```python
from build123d import *

# Parameters (mm, degrees)
SALIENTE_EXTRUIR1_DEPTH = 111
SALIENTE_EXTRUIR2_DEPTH = 6
CROQUIS3_W              = 20
CROQUIS3_H              = 5
SALIENTE_EXTRUIR3_DEPTH = 2
SALIENTE_EXTRUIR4_DEPTH = 6
SALIENTE_EXTRUIR5_DEPTH = 2
CROQUIS6_R              = 2
CORTAR_EXTRUIR1_DEPTH   = 41
CROQUIS7_R              = 4
CORTAR_EXTRUIR2_DEPTH   = 4
CROQUIS9_W              = 16.2
CROQUIS9_H              = 53
CORTAR_EXTRUIR4_DEPTH   = 20
CORTAR_EXTRUIR5_DEPTH   = 119


with BuildPart() as part:
    # Croquis1 → Saliente-Extruir1 (new body)
    with BuildSketch(Plane.XY):
        with BuildLine():
            Line((0, 5), (0, 0))
            Line((0, 0), (28, 0))
            ThreePointArc((28, 0), (29.414213562, 0.585786438), (30, 2))
            Line((30, 2), (30, 13))
            ThreePointArc((30, 13), (29.414213562, 14.414213562), (28, 15))
            Line((28, 15), (0, 15))
            Line((0, 15), (0, 10))
            Line((0, 10), (20, 10))
            Line((20, 10), (20, 5))
            Line((20, 5), (0, 5))
        make_face()
    extrude(amount=SALIENTE_EXTRUIR1_DEPTH)

    # Croquis2 → Saliente-Extruir2 (add)
    with BuildSketch(Plane.XY.offset(111)):
        with BuildLine():
            Line((20, 15), (20, 10))
            Line((20, 10), (20, 5))
            Line((20, 5), (0, 5))
            Line((0, 5), (0, 0))
            Line((0, 0), (28, 0))
            ThreePointArc((28, 0), (29.414213562, 0.585786438), (30, 2))
            Line((30, 2), (30, 13))
            ThreePointArc((30, 13), (29.414213562, 14.414213562), (28, 15))
            Line((28, 15), (20, 15))
        make_face()
    extrude(amount=SALIENTE_EXTRUIR2_DEPTH)

    # Croquis3 → Saliente-Extruir3 (add)
    with BuildSketch(Plane.XY.offset(117)):
        Polygon((20, 10), (20, 15), (11, 15), (0, 15), (0, 10), align=None)
        with BuildLine():
            Line((28, 15), (20, 15))
            Line((20, 15), (20, 10))
            Line((20, 10), (20, 5))
            Line((20, 5), (0, 5))
            Line((0, 5), (0, 0))
            Line((0, 0), (28, 0))
            ThreePointArc((28, 0), (29.414213562, 0.585786438), (30, 2))
            Line((30, 2), (30, 13))
            ThreePointArc((30, 13), (29.414213562, 14.414213562), (28, 15))
        make_face()
        with Locations((10, 7.5)):
            Rectangle(CROQUIS3_W, CROQUIS3_H)
    extrude(amount=SALIENTE_EXTRUIR3_DEPTH)

    # Croquis4 → Saliente-Extruir4 (add)
    with BuildSketch(Plane(origin=(0, 0, 0), x_dir=(-1, 0, 0), z_dir=(0, 0, -1))):
        with BuildLine():
            Line((-20, 5), (-20, 10))
            Line((-20, 10), (-20, 15))
            Line((-20, 15), (-28, 15))
            ThreePointArc((-28, 15), (-29.414213562, 14.414213562), (-30, 13))
            Line((-30, 13), (-30, 2))
            ThreePointArc((-30, 2), (-29.414213562, 0.585786438), (-28, 0))
            Line((-28, 0), (0, 0))
            Line((0, 0), (0, 5))
            Line((0, 5), (-20, 5))
        make_face()
    extrude(amount=SALIENTE_EXTRUIR4_DEPTH)

    # Croquis5 → Saliente-Extruir5 (add)
    with BuildSketch(Plane(origin=(0, 0, -6), x_dir=(-1, 0, 0), z_dir=(0, 0, -1))):
        with BuildLine():
            Line((0, 15), (-28, 15))
            ThreePointArc((-28, 15), (-29.414213562, 14.414213562), (-30, 13))
            Line((-30, 13), (-30, 2))
            ThreePointArc((-30, 2), (-29.414213562, 0.585786438), (-28, 0))
            Line((-28, 0), (0, 0))
            Line((0, 0), (0, 15))
        make_face()
    extrude(amount=SALIENTE_EXTRUIR5_DEPTH)

    # Croquis6 → Cortar-Extruir1 (cut)
    with BuildSketch(Plane.XZ):
        with Locations((5, 24.25)):
            Circle(CROQUIS6_R)
        with Locations((5, 86.75)):
            Circle(CROQUIS6_R)
    extrude(amount=-CORTAR_EXTRUIR1_DEPTH, mode=Mode.SUBTRACT)

    # Croquis7 → Cortar-Extruir2 (cut)
    with BuildSketch(Plane(origin=(0, 0, 0), x_dir=(-1, 0, 0), z_dir=(0, -1, 0))):
        with Locations((-5, -24.25)):
            Circle(CROQUIS7_R)
        with Locations((-5, -86.75)):
            Circle(CROQUIS7_R)
    extrude(amount=-CORTAR_EXTRUIR2_DEPTH, mode=Mode.SUBTRACT)

    # Croquis9 → Cortar-Extruir4 (cut)
    with BuildSketch(Plane.XZ):
        with Locations((8.1, 55.674909876)):
            Rectangle(CROQUIS9_W, CROQUIS9_H)
    extrude(amount=-CORTAR_EXTRUIR4_DEPTH, mode=Mode.SUBTRACT)

    # Croquis10 → Cortar-Extruir5 (cut)
    with BuildSketch(Plane(origin=(0, 0, -8), x_dir=(-1, 0, 0), z_dir=(0, 0, -1))):
        Polygon((-26.910638664, 15), (-28.420130104, 12.506734448), (-23.909345161, 9.909393396), (-20.827352116, 15), align=None)
    extrude(amount=-CORTAR_EXTRUIR5_DEPTH, mode=Mode.SUBTRACT)


solid = part.part
```
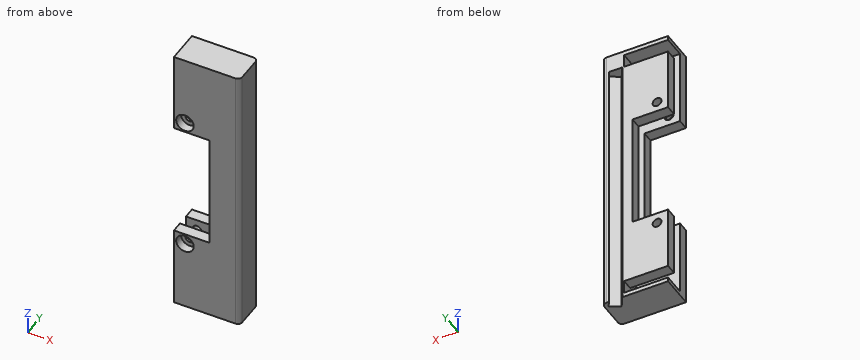
Design review of the part built by this model. Coordinates are the model's own, in mm. Coordinates: 2 decimals unless noted, no trailing zeros. Order: outer loops, then holes, each group sorted by start corner. A loop starts at its lowest first (then second) coordinate and runs counter-clockwise, first axis right, second up. Notation, with made-up numbers: M 59.5,81.5 L 87.5,81.5 A30 cw 87.5,116.5 Z; hole C 57,87 d3. An arc over 180 degrees is marked long. Answer as a JSON object with one key per item and string values. Group by question number.
1) Add section A-A, the plane z = 24.25. Write out the cut boundary in (x, y).
2) Add section C-C, the plane y = 7.75. Write out the cut boundary in (x, z).
3) Add section D-D, the plane x = 5. Count the separate pieces of the cut face and the enclosed holes in it, then the cut area to 3 significant figures.
4) Add section B-B, the plane x = 15. Write out the cut boundary in (y, z).
5) For pin 1 (5 mm diameter, centred on x = 5, z = 24.25, fed in from -Y); pin 2 (4.5 mm diameter, centred on x = 5, z = 86.75, fed in from +Y); pin 3 (4 mm diameter, centred on y = 13, z = 52.5, fed in from -X), all flat-tipped, find the tip position at first contact; note any pin that passes through.
6) Wall thickness on L1, parallel to Z at x = 11.5, y = 10.25; L2, parallel to Z at x = 5, y = 12.85; L3, parallel to Z at x = 5, y = 1: over which ranges is each line inside the solid? List them lowest first.
Computed values:
{
 "1": {"outline": "M 0,0 L 1,0 L 1,4 L 3,4 L 3,5 L 0,5 Z; M 0,10 L 3,10 L 3,15 L 0,15 Z; M 7,4 L 9,4 L 9,0 L 28,0 A2 ccw 30,2 L 30,13 A2 ccw 28,15 L 26.91,15 L 28.42,12.51 L 23.91,9.91 L 20.83,15 L 7,15 L 7,10 L 20,10 L 20,5 L 7,5 Z"},
 "2": {"outline": "M 0,-8 L 30,-8 L 30,119 L 0,119 L 0,117 L 20,117 L 20,-6 L 0,-6 Z"},
 "3": {"separate pieces": "8", "enclosed holes": "0", "area": "588 mm^2"},
 "4": {"outline": "M 0,-8 L 15,-8 L 15,-6 L 5,-6 L 5,29.17 L 0,29.17 Z; M 0,82.17 L 5,82.17 L 5,117 L 15,117 L 15,119 L 0,119 Z; M 10,0 L 15,0 L 15,29.17 L 10,29.17 Z; M 10,82.17 L 15,82.17 L 15,111 L 10,111 Z"},
 "5": {"pin 1": "stops at y = 4", "pin 2": "stops at y = 15", "pin 3": "stops at x = 16.2"},
 "6": {"L1": "z = -8 to -6, 0 to 29.17, 82.17 to 111, 117 to 119", "L2": "z = -8 to -6, 0 to 22.25, 26.25 to 29.17, 82.17 to 84.75, 88.75 to 111, 117 to 119", "L3": "z = -8 to 20.25, 28.25 to 29.17, 82.17 to 82.75, 90.75 to 119"}
}
